The listing builds one solid part. Answer for the finished solid, in the listing's coordinates (mm). Round coordinates to 2 decimals unless told otherwise and drop trailing zeros. Write each loop counter-clockwise with the first axis right and the second up, starting at its lowest first coordinate (ties: lowest second). Pieces come first, ordered by that corner, then holes. Notation, with made-up numbers: M -24.75,23.25 L -9.75,23.25 A25 ccw -9.75,60.25 Z; hole C 55.5,12.5 d5. An arc over 180 degrees is marked long. Put each result on its own line as item: value. Start each with the question number.
```python
from build123d import *

# Parameters (mm, degrees)
BOSS_EXTRUDE1_DEPTH                                 = 3
SKETCH2_R                                           = 6
BOSS_EXTRUDE2_DEPTH                                 = 2
TAP_DRILL_FOR_M3X0_5_TAP1_D                         = 2.6
SKETCH5_R                                           = 2.5
CUT_EXTRUDE1_DEPTH                                  = 35.146742158
CSK_FOR_M3_FLAT_COUNTERSUNK_HEAD_SCREW1_D           = 3.4
CSK_FOR_M3_FLAT_COUNTERSUNK_HEAD_SCREW1_DEPTH       = 6
CSK_FOR_M3_FLAT_COUNTERSUNK_HEAD_SCREW1_CSINK_D     = 6.3
CSK_FOR_M3_FLAT_COUNTERSUNK_HEAD_SCREW1_CSINK_ANGLE = 90
CSK_FOR_M3_FLAT_COUNTERSUNK_HEAD_SCREW1_TIP         = 1.021463052


with BuildPart() as part:
    # Sketch1 → Boss-Extrude1 (new body)
    with BuildSketch(Plane.XY):
        with BuildLine():
            Line((6.492075468, 12.403747664), (25.393424513, 5.987087535))
            ThreePointArc((25.393424513, 5.987087535), (30.969865577, 0.600587203), (26.5781102, -5.788744959))
            Line((26.5781102, -5.788744959), (7.022947864, -12.11107771))
            ThreePointArc((7.022947864, -12.11107771), (-13.996718533, -0.30310114), (6.492075468, 12.403747664))
        make_face()
    extrude(amount=BOSS_EXTRUDE1_DEPTH)

    # Sketch2 → Boss-Extrude2 (add)
    with BuildSketch(Plane.XY.offset(3)):
        with Locations(Location((25, 0, 0), (0, 0, 86.240375256))):
            Circle(SKETCH2_R)
    extrude(amount=BOSS_EXTRUDE2_DEPTH)

    # Tap Drill for M3x0.5 Tap1 (through all)
    with Locations(Plane.XY.offset(5)):
        with Locations((25, 0)):
            Hole(TAP_DRILL_FOR_M3X0_5_TAP1_D / 2)

    # Sketch5 → Cut-Extrude1 (cut, through all)
    with BuildSketch(Plane.XY.offset(3)):
        Circle(SKETCH5_R)
    extrude(amount=-CUT_EXTRUDE1_DEPTH, mode=Mode.SUBTRACT)

    # CSK for M3 Flat Countersunk Head Screw1
    with Locations(Plane.XY.offset(3)):
        with Locations((0, 10), (-10, 0), (0, -10), (10, 0)):
            CounterSinkHole(CSK_FOR_M3_FLAT_COUNTERSUNK_HEAD_SCREW1_D / 2, CSK_FOR_M3_FLAT_COUNTERSUNK_HEAD_SCREW1_CSINK_D / 2, depth=CSK_FOR_M3_FLAT_COUNTERSUNK_HEAD_SCREW1_DEPTH, counter_sink_angle=CSK_FOR_M3_FLAT_COUNTERSUNK_HEAD_SCREW1_CSINK_ANGLE)
            with Locations((0, 0, -(CSK_FOR_M3_FLAT_COUNTERSUNK_HEAD_SCREW1_DEPTH + CSK_FOR_M3_FLAT_COUNTERSUNK_HEAD_SCREW1_TIP / 2))):  # 118° drill point
                Cone(0, CSK_FOR_M3_FLAT_COUNTERSUNK_HEAD_SCREW1_D / 2, CSK_FOR_M3_FLAT_COUNTERSUNK_HEAD_SCREW1_TIP, mode=Mode.SUBTRACT)


solid = part.part
```
Item 1: Consider line 1 along Y through (x, z) = (0, 0.45); line 2 along Y through (x, z) = (1.5, 2.6); line 3 along Z through (x, y) = (2, -3.75). Determine where each line is inside the solid, lowest interval first. Write a range as [from, to].
Item 2: Determine the mould class of faces 1 (the flat face through (4, 0, 0)), 2 (the cylindrical face through (-13.98, -0.71, 1.48)), 3 (the cylindrical face through (8.43, -0.65, 0.76)), 4 (the cylindrical face through (0.37, -11.66, 0.76)) for opening direction Y: released by +Y, released by -Y, zero draft, split by the parting line, or undercut.
Item 3: Flat-ended cylindrical pins translate along their axes: pin 1 (2 mm diameter, centred on x = 25, y = 0, fed in from -Z); pin 2 (4 mm diameter, centred on x = 0, y = 10, fed in from +Z); pin 3 (5.5 mm diameter, centred on x = -10, y = 0, fed in from +Z); pin 4 (3 mm diameter, centred on x = 13.5, y = -10.5, fed in from +Z). Find the tip coordinate at first contact, or state that the pin passes through.
Item 4: Section C-C (z = 0.65) is taken. Give the vertices of the cut face in (x, y), and give its area (3 significant figures).
Item 5: Section A-A (x = 0) is taken. Give the vertices of the cut face in (y, z).
Item 6: Section B-B (y = 0) is taken. Give the vertices of the cut face in (x, z).
Item 7: Section D-D (x = 10) is taken. Give the vertices of the cut face in (y, z), and give its area (3 significant figures).
Output values:
1. line 1: y = [-14, -11.7], [-8.3, -2.5], [2.5, 8.3], [11.7, 14]
1. line 2: y = [-13.92, -12.3], [-7.7, -2], [2, 7.7], [12.3, 13.92]
1. line 3: z = [0, 3]
2. face 1: zero draft
2. face 2: split by the parting line
2. face 3: undercut
2. face 4: undercut
3. pin 1: passes through
3. pin 2: stops at z = 1.85
3. pin 3: stops at z = 2.6
3. pin 4: stops at z = 3
4. outline: M 6.49,12.4 A14 ccw long 7.02,-12.11 L 26.58,-5.79 A6 ccw 25.39,5.99 Z; hole C -10,0 d3.4; hole C 0,0 d5; hole C 0,-10 d3.4; hole C 0,10 d3.4; hole C 10,0 d3.4; hole C 25,0 d2.6
4. area: 822 mm^2
5. outline: M -14,0 L -11.7,0 L -11.7,1.55 L -13.15,3 L -14,3 Z; M -8.3,0 L -2.5,0 L -2.5,3 L -6.85,3 L -8.3,1.55 Z; M 2.5,0 L 8.3,0 L 8.3,1.55 L 6.85,3 L 2.5,3 Z; M 11.7,0 L 14,0 L 14,3 L 13.15,3 L 11.7,1.55 Z
6. outline: M -14,0 L -11.7,0 L -11.7,1.55 L -13.15,3 L -14,3 Z; M -8.3,0 L -2.5,0 L -2.5,3 L -6.85,3 L -8.3,1.55 Z; M 2.5,0 L 8.3,0 L 8.3,1.55 L 6.85,3 L 2.5,3 Z; M 11.7,0 L 23.7,0 L 23.7,5 L 19,5 L 19,3 L 13.15,3 L 11.7,1.55 Z; M 26.3,0 L 31,0 L 31,5 L 26.3,5 Z
7. outline: M -11.15,0 L -1.7,0 L -1.7,1.55 L -3.15,3 L -11.15,3 Z; M 1.7,0 L 11.21,0 L 11.21,3 L 3.15,3 L 1.7,1.55 Z
7. area: 54.8 mm^2
